Autodesk Fusion 360 part; units mm, degrees
sketch "Sketch1" plane through (1.7731, -80, 44.5975) normal (0, -1, 0) x (1, 0, 0)
  circle A0 centre (-18.2269, 40.4025) radius 1
  line L0 (-21.3196, -42.597) -> (-21.3196, 42.597)
  line L1 (93.2269, 42.5973) -> (-81.7731, 42.5973)
  circle A1 centre (18.7731, 40.4025) radius 1
  line L2 (21.3196, -42.597) -> (21.3196, 42.597)
  line L3 (-21.3196, 42.597) -> (20.8249, 42.597)
  line L4 (20.8249, 42.597) -> (20.8249, 38.2081)
  line L5 (20.8249, 38.2081) -> (-21.3196, 38.2081)
  line L6 (-21.3196, 38.2081) -> (-21.3196, 42.597)
  line L7 (-21.3196, 42.597) -> (20.8249, 38.2081) construction
  line L8 (20.8249, 42.597) -> (-21.3196, 38.2081) construction
  point P0 (-0.2473, 40.4025)
extrude "Extrude1" add sketch "Sketch1" along normal blind 2
fillet "Fillet1" radius 1 4 edges at (1.5258, -80, 87.1945) (-19.5465, -80, 85) (1.5258, -80, 82.8055) (22.598, -80, 85)
delete_face "DeleteFace1" 1 faces at (21.938, -80.0596, 84.5216)
fillet "Fillet2" radius 1 2 edges at (1.5258, -82, 87.1945) (1.5258, -82, 82.8055)
Build history of the part. All positions in model axes, mm. Coordinates: 2 decimals unless noted, no trailing zeros. Order: outer loops, then holes, each group sorted by start corner. A loop starts at its lowest first (then second) coordinate and runs counter-clockwise, first axis right, second up. Notation, with made-up numbers: (-24, 48.25) - (-12, 48.25) arc R27 cw to (-12, 78.25) - close; hole circle Ø4 at (68, 75). An arc over 180 degrees is marked (long way). Write item = value, one per line. Start each with the question number.
1) Two-plate mould, pull along Z, no slides. Class faces 1 (the face through (1.23, -81.7, 83.09)), 2 (the face through (21.008, -80.986, 85.887)), 3 (the face through (-15.992, -80.986, 85.887)), 4 (the face through (1.23, -80.3, 86.91)): pulls with the +Z half, pulls with the -Z half, needs draft (parallel to the pull), parting line crosses it, or undercut.
2) Saw through at D-D on z = 83.35. Write the cut outline in (x, y), then the cut area to 3 significant figures.
3) Saw through at A-A on z = 85. Write the cut outline in (x, y), then the cut area to 3 significant figures.
4) Wall check: line 1 along X through (y, z) = (-80.3, 85.65); line 2 along X through (y, z) = (-81.3, 85); line 3 along Y through (x, z) = (-7.5, 86.3). Give the ranges that are in metal, low to high. Write a range as from..to.
5) Saw through at C-C on y = -81.4. Write the cut outline in (x, z).
From the geometry:
q1.face_1 = pulls with the -Z half
q1.face_2 = undercut
q1.face_3 = undercut
q1.face_4 = pulls with the +Z half
q2.outline = (-19.55, -81.89) - (22.6, -81.89) - (22.6, -80.11) - (-19, -80.11) arc R1 ccw to (-19.55, -81) - close
q2.area = 74.9 mm^2
q3.outline = (-19.55, -82) - (-17.45, -82) - (-17.45, -80) - (-18.55, -80) arc R1 ccw to (-19.55, -81) - close; (-15.45, -82) - (19.55, -82) - (19.55, -80) - (-15.45, -80) - close; (21.55, -82) - (22.6, -82) - (22.6, -80) - (21.55, -80) - close
q3.area = 76.1 mm^2
q4.line_1 = -19.26..-17.21, -15.69..19.79, 21.31..22.6
q4.line_2 = -19.55..-17.45, -15.45..19.55, 21.55..22.6
q4.line_3 = -81.99..-80.01
q5.outline = (-19.55, 82.89) - (22.6, 82.89) - (22.6, 87.11) - (-19.55, 87.11) - close; hole circle Ø2 at (-16.45, 85); hole circle Ø2 at (20.55, 85)
